Work out the finished part from the listing and answer in its coordinate system (mm). A direction names the side the tool comes from. Give positions to 0.01 mm unless a question says otherwise; leave off trailing zeros. Write each loop counter-clockwise with the first axis right and the second up, starting at its lowest first coordinate (ties: lowest second). Pieces come first, ordered by that corner, then holes. Notation, with made-up numbers: (-10.5, -24.5) -> (-6.5, -24.5) arc R31 cw to (-6.5, 0.5) -> close; hole circle Ø6 at (-16, -15.5). An arc over 180 degrees is marked (long way). Use a Markdown table: item, result. Add a question column.
Q1. Section D-D, the plane y = 9.5 is taken. Give the vertices of the cut face in (x, z).
Q2. Consider line 1 (Z direction, x = 9.25, y = 17); line 2 (X direction, y = 0.4, z = 0); line 3 (Y direction, x = -5.5, z = -2.25). Determine where each line is inside the solid, lowest interval first.
Q3. Each of these flat-tipped pins is pushed along its axis until it touches: pin 1 Ø12 at (x, y) = (0.5, 22) entering from +Z; pin 2 Ø5 at (x, z) = (4, 0.5) entering from +Y; pin 3 Ø1.9 at (x, z) = (10, -0.5) entering from -Y. Where does it stop, or does it pass through?
Q4. For a pull along Z with two mould halves and no side action, classify faces 1 (the face through (-9, 10, 5)), 2 (the face through (9.6, 14.9, -3.2)), 3 (the face through (8.92, 0.38, 0.07)), 4 (the face through (-9.7, 14.9, 3.2)) as pulls with the +Z half, pulls with the -Z half, needs draft (parallel to the pull), parting line crosses it, or undercut.
Q5. Section B-B, the plane z = 0 is taken. State how many separate pieces and enclosed holes the cut face has, plus the area to 3 significant figures.
Q6. Section A-A, the plane x = 0 is taken. Give the vertices of the cut face in (y, z), plus the area to 3 significant figures.
Q7. For faces 5 (the face through (9.64, 22.32, -3.21)), 6 (the face through (-9, 10, -5)), 7 (the face through (8.8, 23, 0)), determine the directions among +Z, -Z, +X, -X, +Y, -Y from which every point of the face is accessible in a straight line to the end or side of a thin tool.
Q8. Section C-C, the plane y = 20.75 is taken. Give the vertices of the cut face in (x, z), plus the area to 3 significant figures.
from build123d import *

# Parameters (mm, degrees)
SALIENTE_EXTRUIR1_DEPTH = 5
CROQUIS2_R              = 4.5
CORTAR_EXTRUIR1_DEPTH   = 28.257564023
CROQUIS3_W              = 7
CROQUIS3_H              = 8
CORTAR_EXTRUIR2_DEPTH   = 33.767740179
REDONDEO1_R             = 2
REDONDEO2_R             = 1


with BuildPart() as part:
    # Croquis1 → Saliente-Extruir1 (new, symmetric)
    with BuildSketch(Plane.XY):
        with BuildLine():
            Line((-8.8, 24.652074892), (-10.5, 24.652074892))
            Line((-10.5, 24.652074892), (-10.5, 12.723760553))
            ThreePointArc((-10.5, 12.723760553), (-10.498289984, 12.652156614), (-10.493163835, 12.580715934))
            Line((-10.493163835, 12.580715934), (-9.417931151, 1.356955381))
            ThreePointArc((-9.417931151, 1.356955381), (-8.933586693, 0.389917361), (-7.924767316, 0))
            Line((-7.924767316, 0), (7.924767316, 0))
            ThreePointArc((7.924767316, 0), (8.933586693, 0.389917361), (9.417931151, 1.356955381))
            Line((9.417931151, 1.356955381), (10.493163835, 12.580715934))
            ThreePointArc((10.493163835, 12.580715934), (10.498289984, 12.652156614), (10.5, 12.723760553))
            Line((10.5, 12.723760553), (10.5, 24.652074892))
            Line((10.5, 24.652074892), (8.8, 24.652074892))
            Line((8.8, 24.652074892), (8.8, 12.739594081))
            ThreePointArc((8.8, 12.739594081), (8.798289984, 12.667990142), (8.793163835, 12.596549461))
            Line((8.793163835, 12.596549461), (7.839995893, 2.646955381))
            ThreePointArc((7.839995893, 2.646955381), (7.355651435, 1.679917361), (6.346832058, 1.29))
            Line((6.346832058, 1.29), (-6.346832058, 1.29))
            ThreePointArc((-6.346832058, 1.29), (-7.355651435, 1.679917361), (-7.839995893, 2.646955381))
            Line((-7.839995893, 2.646955381), (-8.793163835, 12.596549461))
            ThreePointArc((-8.793163835, 12.596549461), (-8.798289984, 12.667990142), (-8.8, 12.739594081))
            Line((-8.8, 12.739594081), (-8.8, 24.652074892))
        make_face()
    extrude(amount=SALIENTE_EXTRUIR1_DEPTH, both=True)

    # Croquis2 → Cortar-Extruir1 (cut, through all)
    with BuildSketch(Plane.XZ):
        with Locations(Location((0, 0, 0), (0, 0, 270))):
            Circle(CROQUIS2_R)
    extrude(amount=-CORTAR_EXTRUIR1_DEPTH, mode=Mode.SUBTRACT)

    # Croquis3 → Cortar-Extruir2 (cut, through all)
    with BuildSketch(Plane(origin=(10.5, 0, 0), x_dir=(0, 0, -1), z_dir=(1, 0, 0))):
        with Locations((0, 18.616395413)):
            Rectangle(CROQUIS3_W, CROQUIS3_H)
    extrude(amount=-CORTAR_EXTRUIR2_DEPTH, mode=Mode.SUBTRACT)

    # Redondeo1
    redondeo1_edges = [part.edges().sort_by_distance(p)[0] for p in [
        (9.65, 24.652074892, -5),
        (-9.65, 24.652074892, -5),
        (9.65, 24.652074892, 5),
        (-9.65, 24.652074892, 5),
    ]]
    fillet(redondeo1_edges, radius=REDONDEO1_R)

    # Redondeo2
    redondeo2_edges = [part.edges().sort_by_distance(p)[0] for p in [
        (-9.65, 22.616395413, -3.5),
        (9.65, 22.616395413, -3.5),
        (-9.65, 14.616395413, -3.5),
        (9.65, 14.616395413, -3.5),
        (-9.65, 14.616395413, 3.5),
        (9.65, 14.616395413, 3.5),
        (-9.65, 22.616395413, 3.5),
        (9.65, 22.616395413, 3.5),
    ]]
    fillet(redondeo2_edges, radius=REDONDEO2_R)


solid = part.part
Result set:
| question | item | result |
|---|---|---|
| 1 | outline | (-10.2, -5) -> (-8.5, -5) -> (-8.5, 5) -> (-10.2, 5) -> close; (8.5, -5) -> (10.2, -5) -> (10.2, 5) -> (8.5, 5) -> close |
| 2 | line 1 | z = -5 to -3.5, 3.5 to 5 |
| 2 | line 2 | x = -8.94 to -4.5, 4.5 to 8.94 |
| 2 | line 3 | y = 0 to 1.29 |
| 3 | pin 1 | passes through |
| 3 | pin 2 | stops at y = 1.3 |
| 3 | pin 3 | stops at y = 0.51 |
| 4 | face 1 | pulls with the +Z half |
| 4 | face 2 | undercut |
| 4 | face 3 | needs draft |
| 4 | face 4 | undercut |
| 5 | separate pieces | 4 |
| 5 | enclosed holes | 0 |
| 5 | area | 64.8 mm2 |
| 6 | outline | (0, -5) -> (1.29, -5) -> (1.29, -4.5) -> (0, -4.5) -> close; (0, 4.5) -> (1.29, 4.5) -> (1.29, 5) -> (0, 5) -> close |
| 6 | area | 1.29 mm2 |
| 7 | face 5 | +X, -X |
| 7 | face 6 | -Z, +X, -X, +Y, -Y |
| 7 | face 7 | +Z, -Z, +Y |
| 8 | outline | (-10.5, -5) -> (-8.8, -5) -> (-8.8, -3.5) -> (-10.5, -3.5) -> close; (-10.5, 3.5) -> (-8.8, 3.5) -> (-8.8, 5) -> (-10.5, 5) -> close; (8.8, -5) -> (10.5, -5) -> (10.5, -3.5) -> (8.8, -3.5) -> close; (8.8, 3.5) -> (10.5, 3.5) -> (10.5, 5) -> (8.8, 5) -> close |
| 8 | area | 10.2 mm2 |
